Autodesk Inventor part; units mm, degrees
ref_plane "YZ Plane" through (0, 0, 0) normal (1, 0, 0) x (0, 1, 0)
ref_plane "XZ Plane" through (0, 0, 0) normal (0, 1, 0) x (-1, 0, 0)
ref_plane "XY Plane" through (0, 0, 0) normal (0, 0, 1) x (1, 0, 0)
sketch "Sketch1" plane through (0, 0, 0) normal (1, 0, 0) x (0, 1, 0)
  line L0 (-10, 10) -> (10, 10)
  line L1 (10, 10) -> (10, -10)
  line L2 (10, -10) -> (-10, -10)
  line L3 (-10, -10) -> (-10, 10)
  line L4 (-10, 10) -> (10, -10) construction
  line L5 (10, 10) -> (-10, -10) construction
  line L6 (7, -7) -> (7, 7)
  line L7 (7, 7) -> (-7, 7)
  line L8 (-7, 7) -> (-7, -7)
  line L9 (-7, -7) -> (7, -7)
  point P0 (0, 0)
  dimension "d0" = 20
  dimension "d1" = 20
  dimension "d2" = 3
extrude "Extrusion1" add sketch "Sketch1" along normal blind 409
properties part number "2020 Extrusion Base"
Work out the finished part from the listing and answer in its coordinate system (mm). A direction names the side the tool comes from. Give positions to 0.01 mm unless a question says otherwise; leave off trailing zeros. Order: outer loops, then holes, each group sorted by start corner. A loop starts at its lowest first (then second) coordinate and runs counter-clockwise, first axis right, second up. Notation, with made-up numbers: (44.25, -32.75) -> (53.25, -32.75) arc R22 ccw to (53.25, -14.75) -> close; hole circle Ø9 at (44, 20). An arc over 180 degrees is marked (long way). One line per item, written item: value.
Item 1: Find section C-C, the plane x = 97. Give the vertices of the cut face in (y, z), plus the area to 3 significant figures.
Answer sheet:
outline: (-10, -10) -> (10, -10) -> (10, 10) -> (-10, 10) -> close; hole (-7, -7) -> (7, -7) -> (7, 7) -> (-7, 7) -> close
area: 204 mm²
Item 2: Determine the mould class of faces 1 (the flat face through (409, -9, 0)), 2 (the flat face through (202, 0, 10)), 3 (the flat face through (202, 7, 0)) for opening direction Z: released by +Z, released by -Z, zero draft, split by the parting line, or undercut.
Answer sheet:
face 1: zero draft
face 2: released by +Z
face 3: undercut
Item 3: A straight line is drawn through the part: probe 1 along Y at (x, z) = (292, 1). Find the intervals that lie inside material, in ascending order.
Answer sheet:
probe 1: -10 to -7, 7 to 10
Item 4: A tool of negligible diameter and unlimited length cuts with its end or side. For faces 4 (the flat face through (202, 0, -7)), 5 (the flat face through (202, 0, -10)), from which of +Z, -Z, +X, -X, +Y, -Y can it reach the whole face along a straight path? Write none if from no direction.
Answer sheet:
face 4: +X, -X
face 5: -Z, +X, -X, +Y, -Y
Item 5: Find section A-A, the plane y = 1.5. Give the vertices of the cut face in (x, z).
Answer sheet:
outline: (0, -10) -> (409, -10) -> (409, -7) -> (0, -7) -> close; (0, 7) -> (409, 7) -> (409, 10) -> (0, 10) -> close
